Source: CAD feature listing. Evaluate the final solid. Frame: model axes, mm. A direction names the side the tool comes from. Give positions to 0.01 mm unless a question says otherwise; leave off trailing zeros. Loops run counter-clockwise (first coordinate to the right, second up) from the corner with the lowest first, then second, coordinate; pieces in that order, holes last. Notation, with made-up numbers: (23.25, -38.5) -> (67.25, -38.5) arc R12 ccw to (67.25, -17.5) -> close; hole circle Ø8 at (-4.5, -5). An arc over 180 degrees is marked (long way). Return JSON: item names as keys, results as strings. Group by question number.
(1) Pin query (flat end, axial travel): pin 1 (1.6 mm diameter, centred on y = -9.5, z = 9.5, fed in from -X); pin 2 (5 mm diameter, centred on y = -0.5, z = 4, fed in from -X); pin 3 (1 mm diameter, centred on y = -9.5, z = 10, fed in from +X); pin 4 (10 mm diameter, centred on x = -23, y = -4.5, fed in from -Z). Return the tip coordinate at first contact, or that it passes through.
(2) Cut plane C-C on y = 3. Return loops of the section in (x, z).
(3) Cut plane B-B on z = 8.25. Return loops of the section in (x, y).
(4) Access query for faces 1 (the face through (-6.35, -10, 9)), 2 (the face through (60.28, 7.46, 1.66)), 3 (the face through (6.35, -10, 9)), 4 (the face through (-60.28, 7.87, 1.59)), 5 (the face through (0, -7.938, 9)). Directions: +Z, -Z, +X, -X, +Y, -Y. A direction counts if a zero-diameter tool reaches every point of the face in a straight line with its end or side. Return the directions, or none.
(5) Ray query, line 1 (Z direction, x = -19, y = 3.5); line 2 (X direction, y = 9.75, z = 5); line 3 (Y direction, x = -12.5, z = 5.25). Return the intervals inside material, ascending. Write a range as from..to.
Autodesk Inventor part; units mm, degrees
ref_plane "YZ Plane" through (0, 0, 0) normal (1, 0, 0) x (0, 1, 0)
ref_plane "XZ Plane" through (0, 0, 0) normal (0, 1, 0) x (-1, 0, 0)
ref_plane "XY Plane" through (0, 0, 0) normal (0, 0, 1) x (1, 0, 0)
sketch "Sketch1" plane through (0, 0, 0) normal (0, 0, 1) x (1, 0, 0)
  line L0 (-57.15, -11.1125) -> (57.15, -11.1125)
  line L1 (57.15, -11.1125) -> (57.15, 11.1125)
  line L2 (57.15, 11.1125) -> (-57.15, 11.1125)
  line L3 (-57.15, 11.1125) -> (-57.15, -11.1125)
  line L4 (-57.15, -11.1125) -> (57.15, 11.1125) construction
  line L5 (57.15, -11.1125) -> (-57.15, 11.1125) construction
  point P0 (0, 0)
  dimension "d0" = 114.3
  dimension "d14" = 22.225
extrude "Extrusion1" add sketch "Sketch1" along normal blind 6.35
sketch "Sketch2" plane through (57.15, -11.1125, 0) normal (1, 0, 0) x (0, 0, -1)
  circle A0 centre (-3.175, 19.05) radius 1.5875
  line L0 (0, 22.225) -> (-6.35, 22.225)
  point P0 (0, 11.1125)
  dimension "d3" = 3.175
  dimension "d4" = 3.175
extrude "Extrusion2" add sketch "Sketch2" along normal blind 6.35
sketch "Sketch3" plane through (-57.15, -11.1125, 0) normal (-1, 0, 0) x (0, 0, 1)
  circle A0 centre (3.175, 19.05) radius 1.5875
  circle A1 centre (3.175, 19.05) radius 1.5875
  point P0 (0, 11.1125)
extrude "Extrusion3" add sketch "Sketch3" along normal blind 6.35
sketch "Sketch4" plane through (0, 0, 6.35) normal (0, 0, 1) x (1, 0, 0)
  line L0 (-57.15, -11.1125) -> (57.15, -11.1125)
  line L1 (-6.35, -11.1125) -> (6.35, -11.1125)
  line L2 (6.35, -11.1125) -> (6.35, -7.9375)
  line L3 (6.35, -7.9375) -> (-6.35, -7.9375)
  line L4 (-6.35, -7.9375) -> (-6.35, -11.1125)
  line L5 (-57.15, 11.1125) -> (-57.15, -11.1125)
  point P0 (0, 0)
  point P1 (6.35, -11.1125)
  dimension "d9" = 12.7
  dimension "d10" = 3.175
  dimension "d11" = 50.8
extrude "Extrusion4" add sketch "Sketch4" along normal blind 6.35
fillet "Fillet1" radius 3.175 2 edges at (0, 11.1125, 6.35) (0, 11.1125, 0)
properties part number "Door"
Answers:
{
 "1": {"pin 1": "x = -6.35", "pin 2": "x = -57.15", "pin 3": "x = 6.35", "pin 4": "z = 0"},
 "2": {"outline": "(-57.15, 0) -> (57.15, 0) -> (57.15, 6.35) -> (-57.15, 6.35) -> close"},
 "3": {"outline": "(-6.35, -11.11) -> (6.35, -11.11) -> (6.35, -7.94) -> (-6.35, -7.94) -> close"},
 "4": {"face 1": "+Z, -X, +Y, -Y", "face 2": "+X", "face 3": "+Z, +X, +Y, -Y", "face 4": "-X", "face 5": "+Z, +X, -X, +Y"},
 "5": {"line 1": "0..6.35", "line 2": "-57.15..57.15", "line 3": "-11.11..10.34"}
}
